Read the model definition and answer for the solid it produces. Units are mm, in the model's axes. Face numbers are marked on the shaded views. Coordinates: 2 decimals unless noted, no trailing zeros. Write each loop counter-clockwise with the first axis right and the second up, starting at its lowest first coordinate (ties: lowest second). Pieces come first, ordered by that corner, then holes.
(1) The part is cut by section A-A, the plane y = 17. Determine the outline of the cut face in (x, z).
(2) The part is cut by section B-B, the plane x = 335. Determine the outline of the cut face in (y, z), and give its area (3 significant figures).
(3) The part is cut by section C-C, the plane y = 5. Determine the outline of the cut face in (x, z), and give its area (3 significant figures).
(4) Determine the mould class of the marked faces 1, 2, 3 and 4 for opening direction Z: pulls with the +Z half, pulls with the -Z half, needs draft (parallel to the pull), parting line crosses it, or undercut.
(5) The part is cut by section D-D, the plane x = 328.25. Determine the outline of the cut face in (y, z), and give its area (3 significant figures).
(6) Straight lines are drawn through the part: line 1 along X through (y, z) = (5, 142.25); line 2 along X through (y, z) = (17, 19.75); line 3 along Z through (x, y) = (317.75, 5.25). For each, find the intervals that lie inside material, in ascending order.
(7) Given pin 1 (6 mm diameter, centred on x = 335.5, z = 45, fed in from +Y); pin 2 (5 mm diameter, centred on y = 3.5, z = 94.5, fed in from -X), each flat-ended and moving along its own axis, determine where each tip first touches the part or whether it passes through.
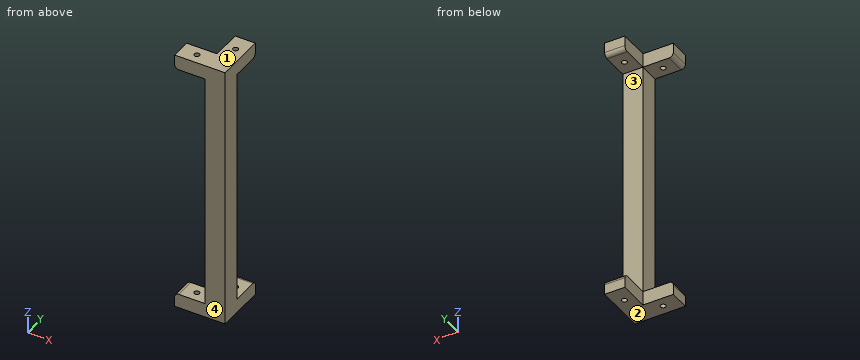
```python
from build123d import *

# Parameters (mm, degrees)
CYLINDER014_R          = 1.3
CYLINDER014_DEPTH      = 146
CYLINDER013_R          = 1.3
CYLINDER013_DEPTH      = 146
BOX072_W               = 10
BOX072_H               = 10
BOX072_DEPTH           = 132
BOX076_W               = 15
BOX076_H               = 10
BOX076_DEPTH           = 7
BOX074_W               = 10
BOX074_H               = 15
BOX074_DEPTH           = 7
BOX075_W               = 10
BOX075_H               = 15
BOX075_DEPTH           = 7
BOX073_W               = 15
BOX073_H               = 10
BOX073_DEPTH           = 7
FILLET002_R            = 2
CUT027_PLACEMENT_ANGLE = 90


with BuildPart() as cilindro014:
    # Cylinder014 → Cylinder014 (new body)
    with BuildSketch(Plane(origin=(5, 17, 8), x_dir=(1, 0, 0), z_dir=(0, 0, 1))):
        Circle(CYLINDER014_R)
    extrude(amount=CYLINDER014_DEPTH)


with BuildPart() as cilindro013:
    # Cylinder013 → Cylinder013 (new body)
    with BuildSketch(Plane(origin=(17, 5, 8), x_dir=(1, 0, 0), z_dir=(0, 0, 1))):
        Circle(CYLINDER013_R)
    extrude(amount=CYLINDER013_DEPTH)


with BuildPart() as cubo035:
    # Box072 → Box072 (new body)
    with BuildSketch(Plane.XY.offset(15)):
        with Locations((5, 5)):
            Rectangle(BOX072_W, BOX072_H)
    extrude(amount=BOX072_DEPTH)


with BuildPart() as cubo039:
    # Box076 → Box076 (new body)
    with BuildSketch(Plane(origin=(10, 0, 140), x_dir=(1, 0, 0), z_dir=(0, 0, 1))):
        with Locations((7.5, 5)):
            Rectangle(BOX076_W, BOX076_H)
    extrude(amount=BOX076_DEPTH)


with BuildPart() as cubo037:
    # Box074 → Box074 (new body)
    with BuildSketch(Plane(origin=(0, 10, 15), x_dir=(1, 0, 0), z_dir=(0, 0, 1))):
        with Locations((5, 7.5)):
            Rectangle(BOX074_W, BOX074_H)
    extrude(amount=BOX074_DEPTH)


with BuildPart() as cubo038:
    # Box075 → Box075 (new body)
    with BuildSketch(Plane(origin=(0, 10, 140), x_dir=(1, 0, 0), z_dir=(0, 0, 1))):
        with Locations((5, 7.5)):
            Rectangle(BOX075_W, BOX075_H)
    extrude(amount=BOX075_DEPTH)


with BuildPart() as obj1:
    # Box073 → Box073 (new body)
    with BuildSketch(Plane(origin=(10, 0, 15), x_dir=(1, 0, 0), z_dir=(0, 0, 1))):
        with Locations((7.5, 5)):
            Rectangle(BOX073_W, BOX073_H)
    extrude(amount=BOX073_DEPTH)

    # Fusion010: union Cubo035, Cubo039, Cubo037, Cubo038
    add(cubo035.part)
    add(cubo039.part)
    add(cubo037.part)
    add(cubo038.part)

    # Fillet002
    fillet002_edges = [obj1.edges().sort_by_distance(p)[0] for p in [
        (25, 5, 22),
        (25, 5, 140),
        (5, 25, 22),
        (5, 25, 140),
    ]]
    fillet(fillet002_edges, radius=FILLET002_R)

    # Cut028: cut Cilindro013
    add(cilindro013.part, mode=Mode.SUBTRACT)

    # Cut027: cut Cilindro014
    add(cilindro014.part, mode=Mode.SUBTRACT)


with BuildPart() as obj1_1:
    # Cut027 placement: moved
    add(obj1.part.moved(Location((340, 0, 0))).rotate(Axis((340, 0, 0), (0, 0, 1)), CUT027_PLACEMENT_ANGLE))


solid = obj1_1.part
```
Computed:
1. outline: (330, 15) - (333.7, 15) - (333.7, 22) - (330, 22) - close; (330, 140) - (333.7, 140) - (333.7, 147) - (330, 147) - close; (336.3, 15) - (340, 15) - (340, 22) - (336.3, 22) - close; (336.3, 140) - (340, 140) - (340, 147) - (336.3, 147) - close
2. outline: (0, 15) - (15.7, 15) - (15.7, 22) - (10, 22) - (10, 140) - (15.7, 140) - (15.7, 147) - (0, 147) - close; (18.3, 15) - (25, 15) - (25, 20) arc R2 ccw to (23, 22) - (18.3, 22) - close; (18.3, 140) - (23, 140) arc R2 ccw to (25, 142) - (25, 147) - (18.3, 147) - close
2. area: 1,490 mm2
3. outline: (315, 15) - (321.7, 15) - (321.7, 22) - (317, 22) arc R2 ccw to (315, 20) - close; (315, 142) arc R2 ccw to (317, 140) - (321.7, 140) - (321.7, 147) - (315, 147) - close; (324.3, 15) - (340, 15) - (340, 147) - (324.3, 147) - (324.3, 140) - (330, 140) - (330, 22) - (324.3, 22) - close
3. area: 1,490 mm2
4. face 1: pulls with the +Z half
4. face 2: pulls with the -Z half
4. face 3: undercut
4. face 4: needs draft
5. outline: (0, 15) - (10, 15) - (10, 22) - (0, 22) - close; (0, 140) - (10, 140) - (10, 147) - (0, 147) - close
5. area: 140 mm2
6. line 1: x = 315 to 321.7, 324.3 to 340
6. line 2: x = 330 to 333.7, 336.3 to 340
6. line 3: z = 15 to 22, 140 to 147
7. pin 1: stops at y = 10
7. pin 2: stops at x = 330
